```python
from build123d import *

# Parameters (mm, degrees)
SKETCH_R        = 20
PAD_DEPTH       = 6.5
SKETCH001_R     = 33
SKETCH001_R_2   = 20
PAD001_DEPTH    = 3
SKETCH002_R     = 3.5
POCKET_DEPTH    = 5
SKETCH003_R     = 31
SKETCH003_R_2   = 23
POCKET001_DEPTH = 2
SKETCH004_R     = 17.5
SKETCH004_R_2   = 12.5
POCKET002_DEPTH = 3.5
CHAMFER_SIZE    = 1


with BuildPart() as part:
    # Sketch → Pad (new body)
    with BuildSketch(Plane.XY):
        Circle(SKETCH_R)
        Polygon((4.907477, 8.5), (-4.907477, 8.5), (-9.814955, 0), (-4.907477, -8.5), (4.907477, -8.5), (9.814955, 0), align=None, mode=Mode.SUBTRACT)
    extrude(amount=PAD_DEPTH)

    # Sketch001 (on Face9 of Pad) → Pad001 (join)
    with BuildSketch(Plane.XY.offset(6.5)):
        Circle(SKETCH001_R)
        Circle(SKETCH001_R_2, mode=Mode.SUBTRACT)
    extrude(amount=-PAD001_DEPTH)

    # Sketch002 (on Face3 of Pad001) → Pocket (cut)
    with BuildSketch(Plane(origin=(0, 0, 3.5), x_dir=(1, 0, 0), z_dir=(0, 0, -1))):
        with Locations((0, 26.5)):
            Circle(SKETCH002_R)
        with Locations((18.73833, 18.73833)):
            Circle(SKETCH002_R)
        with Locations((26.5, 0)):
            Circle(SKETCH002_R)
        with Locations((18.73833, -18.73833)):
            Circle(SKETCH002_R)
        with Locations((0, -26.5)):
            Circle(SKETCH002_R)
        with Locations((-18.73833, -18.73833)):
            Circle(SKETCH002_R)
        with Locations((-26.5, 0)):
            Circle(SKETCH002_R)
        with Locations((-18.73833, 18.73833)):
            Circle(SKETCH002_R)
    extrude(amount=-POCKET_DEPTH, mode=Mode.SUBTRACT)

    # Sketch003 (on Face3 of Pocket) → Pocket001 (cut)
    with BuildSketch(Plane(origin=(0, 0, 3.5), x_dir=(1, 0, 0), z_dir=(0, 0, -1))):
        Circle(SKETCH003_R)
        Circle(SKETCH003_R_2, mode=Mode.SUBTRACT)
    extrude(amount=-POCKET001_DEPTH, mode=Mode.SUBTRACT)

    # Sketch004 (on Face2 of Pocket001) → Pocket002 (cut)
    with BuildSketch(Plane(origin=(0, 0, 0), x_dir=(1, 0, 0), z_dir=(0, 0, -1))):
        Circle(SKETCH004_R)
        Circle(SKETCH004_R_2, mode=Mode.SUBTRACT)
    extrude(amount=-POCKET002_DEPTH, mode=Mode.SUBTRACT)

    # Chamfer
    chamfer_edges = [part.edges().sort_by_distance(p)[0] for p in [
        (7.361216, 4.25, 0),
        (0, 8.5, 0),
        (-7.361216, 4.25, 0),
        (-7.361216, -4.25, 0),
        (0, -8.5, 0),
        (7.361216, -4.25, 0),
    ]]
    chamfer(chamfer_edges, length=CHAMFER_SIZE)


solid = part.part
```
Input: part model. Units: mm. Frame: model coordinates. A direction names the side the tool comes from. Round coordinates to 2 decimals unless told otherwise and drop trailing zeros. Loops run counter-clockwise (first coordinate to the right, second up) from the corner with the lowest first, then second, coordinate; pieces in that order, holes last. Notation, with made-up numbers: M 49,50.5 L 95,50.5 A28 cw 95,86.5 Z; hole C 37,2 d7. An arc over 180 degrees is marked long. Answer in a Markdown table with one row per item. Add a question column.
1. Section B-B (y = 26.5). Output: boundary loops of the cut face in (x, z), and give its area (3 significant figures).
2. Section D-D (y = -13.5). Output: boundary loops of the cut face in (x, z), and give its area (3 significant figures).
3. Mould query, pull axis Y, two halves, no side actions, for faces 4 (the face through (-23.16, -1.05, 5.99)), 5 (the face through (-7, 19, 3.5)), 6 (the face through (-4.336, -19.524, 1.726)). Classes: released by +Y, released by -Y, zero draft, split by the parting line, or undercut.
4. Section A-A (z = 2.5). Output: boundary loops of the cut face in (x, y).
5. Set-up query: faces 1 (the face through (7.762, -4.57, 0.493)), 2 (the face through (0, -8.5, 4)), 3 (the face through (0, -18, 0)). Return all of +Z, -Z, +X, -X, +Y, -Y with unobstructed straight access to the full face (end or side cutting, diameter ignored); none if empty.
6. Ray query, probe 1 along Y at (x, z) = (0, 4.9); probe 2 along X at (y, z) = (-13.5, 3.75); probe 3 along Y at (x, z) = (-4.5, 2.5). Return the intervals inside material, ascending.
7. Contact query for flat-ended pins moving along their axis: pin 1 (1.5 mm diameter, centred on y = 19.5, z = 5.5, fed in from +X); pin 2 (3 mm diameter, centred on x = 13, z = 5.5, fed in from -Y); pin 3 (3 mm diameter, centred on y = -13.5, z = 5.5, fed in from +X). Output: stop coordinate, or through.
Values follow:
| question | item | result |
|---|---|---|
| 1 | outline | M -19.67,3.5 L -16.09,3.5 L -16.09,5.5 L -3.5,5.5 L -3.5,6.5 L -19.67,6.5 Z; M 3.5,5.5 L 16.09,5.5 L 16.09,3.5 L 19.67,3.5 L 19.67,6.5 L 3.5,6.5 Z |
| 1 | area | 46.7 mm^2 |
| 2 | outline | M -30.11,3.5 L -27.91,3.5 L -27.91,5.5 L -18.62,5.5 L -18.62,3.5 L -14.76,3.5 L -14.76,0 L -11.14,0 L -11.14,3.5 L 11.14,3.5 L 11.14,0 L 14.76,0 L 14.76,3.5 L 18.62,3.5 L 18.62,5.5 L 27.91,5.5 L 27.91,3.5 L 30.11,3.5 L 30.11,6.5 L -30.11,6.5 Z |
| 2 | area | 169 mm^2 |
| 3 | face 4 | undercut |
| 3 | face 5 | zero draft |
| 3 | face 6 | split by the parting line |
| 4 | outline | C 0,0 d40; C 0,0 d25; hole C 0,0 d35; hole M -9.81,0 L -4.91,-8.5 L 4.91,-8.5 L 9.81,0 L 4.91,8.5 L -4.91,8.5 Z |
| 5 | face 1 | -Z |
| 5 | face 2 | +Z, -Z |
| 5 | face 3 | -Z, +X, -X, +Y, -Y |
| 6 | probe 1 | -33 to -31, -23 to -8.5, 8.5 to 23, 31 to 33 |
| 6 | probe 2 | -30.11 to -27.91, -18.62 to 18.62, 27.91 to 30.11 |
| 6 | probe 3 | -19.49 to -16.91, -11.66 to -8.5, 8.5 to 11.66, 16.91 to 19.49 |
| 7 | pin 1 | x = 27.16 |
| 7 | pin 2 | y = -30.93 |
| 7 | pin 3 | x = 30.74 |
